Answer from the drawing. Dimensions are ordinates in mm from the lowest x, y and z of the part. A direction names the side the tool comes from. Give positions to 0.01 mm unless a question says otherwise; leave off trailing zeros. Order: outer loops, then holes, each group sorted by start corner. A loop starts at its lowest first (then second) coordinate and runs counter-clockwise, first axis right, second up. Notation, with made-up numbers: (6.5, 72.25) - (10.5, 72.25) arc R8 ccw to (10.5, 83.25) - close; hole circle Ø7 at (-37, -5.5). An arc over 180 degrees is marked (long way). Write each question's results on one line, items separated by ' | '.
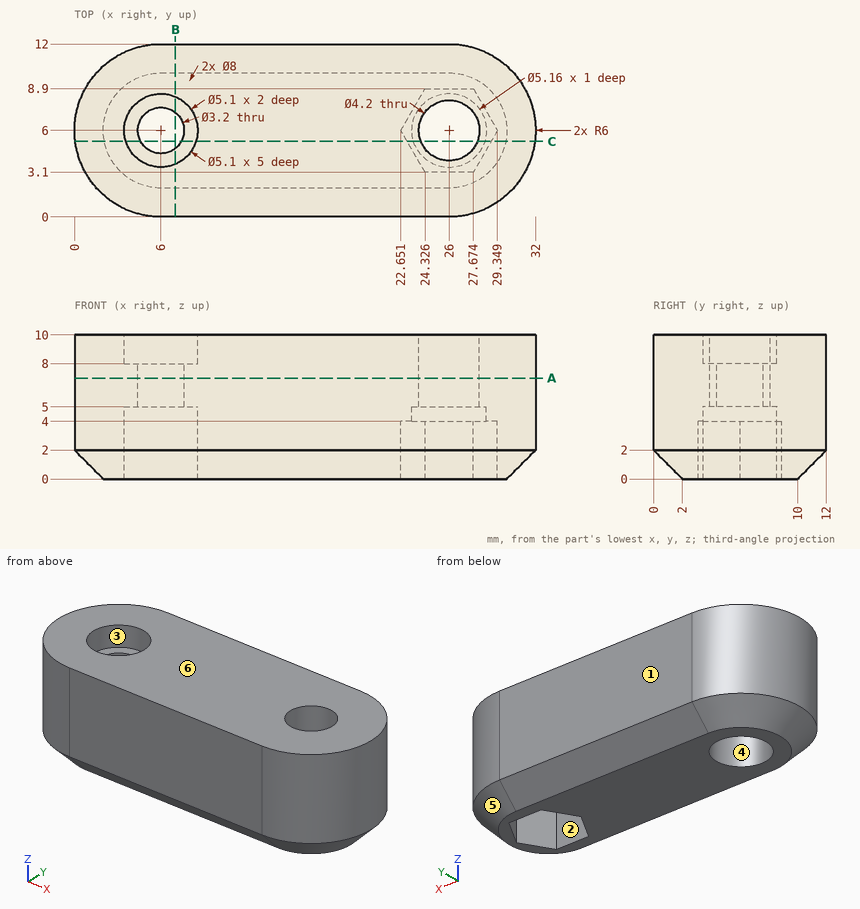
1. Straight lines are drawn through the part: line 1 (Y direction, x = 6, z = 6.45); line 2 (X direction, y = 7, z = 1) (1 decimal); line 3 (X direction, y = 4.5, z = 3). For each, find the intervals that lie inside material, in ascending order. Write a range as [from, to].
Answer list:
line 1: [0, 4.4], [7.6, 12] | line 2: [1.1, 3.7], [8.3, 23.2], [28.8, 30.9] | line 3: [0.19, 3.94], [8.06, 23.52], [28.48, 31.81]
2. A cutting plane is placed at C-C, the plane y = 5.25. State how many separate pieces and enclosed holes the cut face has.
Answer list:
separate pieces: 3 | enclosed holes: 0
3. A cutting plane is placed at A-A, the plane z = 7. Write down the section's boundary in (x, y).
Answer list:
outline: (6, 0) - (26, 0) arc R6 ccw to (26, 12) - (6, 12) arc R6 ccw to start; hole circle Ø3.2 at (6, 6); hole circle Ø4.2 at (26, 6)
4. Given P1, Ø4, axis at x = 6, y = 5.5, coming from the -Z side; P2, Ø1.5, axis at y = 10, z = 7, coming from the -X side; P3, Ø4, axis at x = 6, y = 6, coming from the +Z side, each flat-ended and moving along its own axis, determine where each tip first touches the part or whether it passes through.
Answer list:
P1: z = 5 | P2: x = 0.96 | P3: z = 8
5. A cutting plane is placed at B-B, the plane x = 7. Write down the section's boundary in (y, z) (1 decimal).
Answer list:
outline: (0, 2) - (2, 0) - (3.7, 0) - (3.7, 5) - (4.8, 5) - (4.8, 8) - (3.7, 8) - (3.7, 10) - (0, 10) - close; (7.2, 5) - (8.3, 5) - (8.3, 0) - (10, 0) - (12, 2) - (12, 10) - (8.3, 10) - (8.3, 8) - (7.2, 8) - close
6. Determine the mould class of the marked faces 4, 5 and 6 for opening direction Y: +Y half, -Y half, draft (parallel to the pull), parting line (faces both ways), or undercut.
Answer list:
face 4: undercut | face 5: parting line | face 6: draft
7. A tool of negligible diameter and unlimited length cuts with its end or side. For the marked faces 1, 2 and 3, from which of +Z, -Z, +X, -X, +Y, -Y can it reach the whole face along a straight path? Write none if from no direction.
Answer list:
face 1: +Z, -Z, +X, -X, +Y | face 2: -Z | face 3: +Z
